```python
from build123d import *

# Parameters (mm, degrees)
ESQUISSE1_W             = 41
ESQUISSE1_H             = 41
BOSS_EXTRU_1_DEPTH      = 1.5
ESQUISSE2_W             = 6
ESQUISSE2_H             = 4
BOSS_EXTRU_2_DEPTH      = 1.5
ESQUISSE3_R             = 12.5
ENL_V_MAT_EXTRU_1_DEPTH = 2.5
ESQUISSE4_R             = 16
ENL_V_MAT_EXTRU_2_DEPTH = 0.1
ESQUISSE5_R             = 16
ENL_V_MAT_EXTRU_3_DEPTH = 0.1
CHANFREIN1_SIZE         = 2
CHANFREIN2_SIZE         = 2


with BuildPart() as part:
    # Esquisse1 → Boss.-Extru.1 (new body)
    with BuildSketch(Plane.XY):
        Rectangle(ESQUISSE1_W, ESQUISSE1_H)
    extrude(amount=BOSS_EXTRU_1_DEPTH)

    # Esquisse2 → Boss.-Extru.2 (add)
    with BuildSketch(Plane(origin=(0, 0, 0), x_dir=(-1, 0, 0), z_dir=(0, 0, -1))):
        with Locations((17.5, 22.5)):
            Rectangle(ESQUISSE2_W, ESQUISSE2_H)
        with Locations((-17.5, -22.5)):
            Rectangle(ESQUISSE2_W, ESQUISSE2_H)
        with Locations((17.5, -22.5)):
            Rectangle(ESQUISSE2_W, ESQUISSE2_H)
    extrude(amount=-BOSS_EXTRU_2_DEPTH)

    # Esquisse3 → Enlèv. mat.-Extru.1 (cut, through all)
    with BuildSketch(Plane(origin=(0, 0, 0), x_dir=(-1, 0, 0), z_dir=(0, 0, -1))):
        Circle(ESQUISSE3_R)
    extrude(amount=-ENL_V_MAT_EXTRU_1_DEPTH, mode=Mode.SUBTRACT)

    # Esquisse4 → Enlèv. mat.-Extru.2 (cut)
    with BuildSketch(Plane(origin=(0, 0, 0), x_dir=(-1, 0, 0), z_dir=(0, 0, -1))):
        Circle(ESQUISSE4_R)
    extrude(amount=-ENL_V_MAT_EXTRU_2_DEPTH, mode=Mode.SUBTRACT)

    # Esquisse5 → Enlèv. mat.-Extru.3 (cut)
    with BuildSketch(Plane.XY.offset(1.5)):
        Circle(ESQUISSE5_R)
    extrude(amount=-ENL_V_MAT_EXTRU_3_DEPTH, mode=Mode.SUBTRACT)

    # Chanfrein1
    chanfrein1_edges = [part.edges().sort_by_distance(p)[0] for p in [
        (-20.5, -24.5, 0.75),
    ]]
    chamfer(chanfrein1_edges, length=CHANFREIN1_SIZE)

    # Chanfrein2
    chanfrein2_edges = [part.edges().sort_by_distance(p)[0] for p in [
        (20.5, -24.5, 0.75),
    ]]
    chamfer(chanfrein2_edges, length=CHANFREIN2_SIZE)


solid = part.part
```
Geometry check sheet. Reference: the model listing, model coordinates, mm. A direction names the side the tool comes from. Coordinates: 2 decimals unless noted, no trailing zeros. Order: outer loops, then holes, each group sorted by start corner. A loop starts at its lowest first (then second) coordinate and runs counter-clockwise, first axis right, second up. Notation, with made-up numbers: (40, 64.5) - (58, 64.5) arc R20 ccw to (58, 68.5) - close; hole circle Ø3 at (46.25, 41). An arc over 180 degrees is marked (long way). Answer in a Markdown table with one row per item. Add a question column.
1. Gauge pin test, flat ends, axial feed: pin 1 Ø6 at (x, y) = (-8, 9.5) entering from +Z; pin 2 Ø0.8 at (x, z) = (-7, 0.5) entering from -Y; pin 3 Ø16 at (x, y) = (8, 3) entering from -Z; pin 4 Ø0.8 at (x, z) = (-5, 1) entering from +Y. Record the tip position at first contact, or that the pin passes through.
2. Access from +Z, -Z, +X, -X, +Y, -Y to the whole of each face (thin tool, end or side, straight path). Record for faces 4 (the face through (-10, -8, 1.4)), 5 (the face through (-14.5, 22, 1)), 6 (the face through (-14.5, -23, 1)).
3. Material ranges on L1, parallel to X at y = 0.5, z = 1.2; L2, parallel to X at y = -22, z = 0.85; L3, parallel to Y at x = 0, z = 0.6, recorded low to high. Write a range as [from, to].
4. Section check D-D (x = 17). Enter the section's corners in (y, z), plus the area to 3 significant figures.
5. Draft check along X on faces 1 (the face through (10, -8, 0.1)), 2 (the face through (-20.5, 1, 1)), 3 (the face through (17, -24.5, 1)). Enter one of: +X half, -X half, draft (parallel to the pull), parting line (faces both ways), or undercut.
6. Section check B-B (z = 0.6). Enter the section's corners in (x, y).
7. Section check A-A (x = 0). Enter the section's corners in (y, z), plus the area to 3 significant figures.
Data:
| question | item | result |
|---|---|---|
| 1 | pin 1 | stops at z = 1.4 |
| 1 | pin 2 | stops at y = -20.5 |
| 1 | pin 3 | stops at z = 0 |
| 1 | pin 4 | stops at y = 20.5 |
| 2 | face 4 | +Z |
| 2 | face 5 | +Z, -Z, +X, +Y |
| 2 | face 6 | +Z, -Z, -Y |
| 3 | L1 | x = [-20.5, -12.49], [12.49, 20.5] |
| 3 | L2 | x = [-20.5, -14.5], [14.5, 20.5] |
| 3 | L3 | y = [-20.5, -12.5], [12.5, 20.5] |
| 4 | outline | (-24.5, 0) - (20.5, 0) - (20.5, 1.5) - (-24.5, 1.5) - close |
| 4 | area | 67.5 mm² |
| 5 | face 1 | undercut |
| 5 | face 2 | -X half |
| 5 | face 3 | draft |
| 6 | outline | (-20.5, -22.5) - (-18.5, -24.5) - (-14.5, -24.5) - (-14.5, -20.5) - (14.5, -20.5) - (14.5, -24.5) - (18.5, -24.5) - (20.5, -22.5) - (20.5, 20.5) - (-14.5, 20.5) - (-14.5, 24.5) - (-20.5, 24.5) - close; hole circle Ø25 at (0, 0) |
| 7 | outline | (-20.5, 0) - (-16, 0) - (-16, 0.1) - (-12.5, 0.1) - (-12.5, 1.4) - (-16, 1.4) - (-16, 1.5) - (-20.5, 1.5) - close; (12.5, 0.1) - (16, 0.1) - (16, 0) - (20.5, 0) - (20.5, 1.5) - (16, 1.5) - (16, 1.4) - (12.5, 1.4) - close |
| 7 | area | 22.6 mm² |
